Read the model definition and answer for the solid it produces. Units are mm, in the model's axes. Face numbers are marked on the shaded views. Give positions to 0.01 mm unless a question says otherwise; leave off trailing zeros. Write each loop counter-clockwise with the first axis right and the second up, starting at its lowest first coordinate (ties: lowest second). Pieces come first, ordered by that corner, then holes. Notation, with made-up numbers: (3.5, -33) - (42.5, -33) arc R32 cw to (42.5, -5) - close; hole circle Ø8 at (70, 21). An arc over 180 degrees is marked (long way). Answer as CSV lines item,"result".
Autodesk Inventor part; units mm, degrees
ref_plane "YZ Plane" through (0, 0, 0) normal (1, 0, 0) x (0, 1, 0)
ref_plane "XZ Plane" through (0, 0, 0) normal (0, 1, 0) x (-1, 0, 0)
ref_plane "XY Plane" through (0, 0, 0) normal (0, 0, 1) x (1, 0, 0)
sketch "Sketch1" plane through (0, 0, 0) normal (0, 1, 0) x (-1, 0, 0)
  circle A0 centre (1.143, 0) radius 39 construction
  circle A1 centre (1.143, 0) radius 42
  line L0 (-21.857, 14) -> (-36.857, 14) construction
  line L1 (-36.857, 14) -> (-36.857, 5) construction
  line L2 (-36.857, 5) -> (-21.857, 5) construction
  line L3 (-21.857, 5) -> (-21.857, 14) construction
  line L4 (1.143, 0) -> (-37.857, 0)
  line L5 (0, 0) -> (0, -22) construction
  dimension "d0" = 78
  dimension "d1" = 9
  dimension "d2" = 15
  dimension "d3" = 5
  dimension "d4" = 23
  dimension "d5" = 84
  dimension "d11" = 1.143
extrude "Extrusion1" add sketch "Sketch1" along normal blind 6
fillet "Fillet1" radius 7 1 edges at (40.857, 0, 0)
shell "Shell1" thickness 2 removed faces 1 at (-4.0377, 6, 12.235)
sketch "Sketch2" plane through (-1.143, 2, 0) normal (0, 1, 0) x (1, 0, 0)
  circle A0 centre (-11.303, -22.606) radius 1.95
  circle A1 centre (18.034, 6.223) radius 1.95
  circle A2 centre (-11.303, -22.606) radius 3.5
  circle A3 centre (18.034, 6.223) radius 3.5
  point P0 (1.143, 0)
  dimension "d12" = 3.9
  dimension "d13" = 3.9
  dimension "d14" = 6.223
  dimension "d15" = 16.891
  dimension "d16" = 22.606
  dimension "d17" = 12.446
  dimension "d18" = 7
  dimension "d19" = 7
extrude "Extrusion2" add sketch "Sketch2" along normal blind 5.5
sketch "Sketch3" plane through (-1.143, 2, 0) normal (0, 1, 0) x (1, 0, 0)
  line L0 (7.5, 19.5) -> (-25.5, 19.5) construction
  line L1 (-25.5, 19.5) -> (-25.5, -9.5) construction
  line L2 (-25.5, -9.5) -> (7.5, -9.5) construction
  line L3 (7.5, -9.5) -> (7.5, 19.5) construction
  line L4 (7.5, 19.5) -> (-25.5, -9.5) construction
  line L5 (-25.5, 19.5) -> (7.5, -9.5) construction
  point P0 (1.143, 0)
  point P1 (-9, 5)
  dimension "d22" = 33
  dimension "d23" = 29
sketch "Sketch5" plane through (-1.143, 6, 0) normal (0, 1, 0) x (1, 0, 0)
  line L0 (31.143, -15) -> (45, -15)
  line L1 (45, -15) -> (45, -3)
  line L2 (45, -3) -> (31.143, -3)
  line L3 (31.143, -3) -> (31.143, -15)
  line L4 (1.143, 0) -> (-32, 0) construction
  line L5 (31.143, 15) -> (45, 15)
  line L6 (45, 15) -> (45, 3)
  line L7 (45, 3) -> (31.143, 3)
  line L8 (31.143, 3) -> (31.143, 15)
  line L9 (-5.857, 30) -> (6.143, 30)
  line L10 (6.143, 30) -> (6.143, 46)
  line L11 (6.143, 46) -> (-5.857, 46)
  line L12 (-5.857, 46) -> (-5.857, 30)
  line L13 (-5.857, 30) -> (6.143, 46) construction
  line L14 (6.143, 30) -> (-5.857, 46) construction
  line L15 (-4.873, -22) -> (5.127, -22)
  line L16 (5.127, -22) -> (5.127, -44)
  line L17 (5.127, -44) -> (-4.873, -44)
  line L18 (-4.873, -44) -> (-4.873, -22)
  line L19 (-4.873, -22) -> (5.127, -44) construction
  line L20 (5.127, -22) -> (-4.873, -44) construction
  point P0 (0.143, 38)
  point P1 (0.127, -33)
  dimension "d24" = 3
  dimension "d25" = 12
  dimension "d26" = 30
  dimension "d29" = 1
  dimension "d30" = 12
  dimension "d31" = 1.016
  dimension "d32" = 10
extrude "Extrusion3" cut sketch "Sketch5" against normal up to surface (4 mm away)
mirror "Mirror1" about plane through (0, 0, 0) normal (0, 0, 1) of "Extrusion2"
sketch "Sketch6" plane through (-12.446, 7.5, 22.606) normal (0, 1, 0) x (1, 0, 0)
  circle A0 centre (0, 0) radius 4.9497
  circle A1 centre (29.337, 28.829) radius 1.95
  circle A2 centre (29.337, 28.829) radius 4.3979
  point P0 (12.446, 22.606)
extrude "Extrusion4" cut sketch "Sketch6" against normal up to surface (5.5 mm away) contours A0 | A1 | A2
properties part number "Case top"
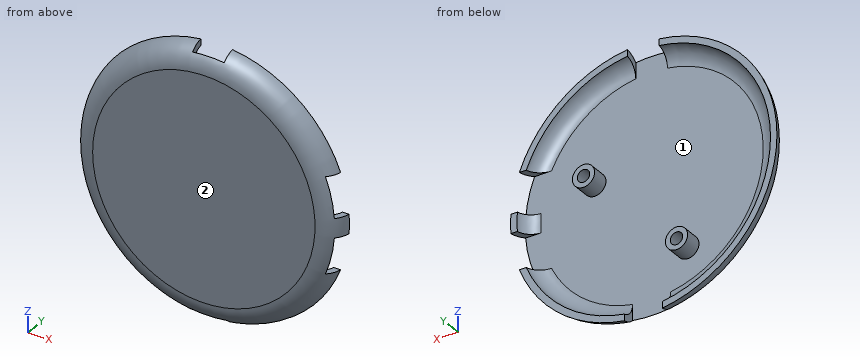
(1) A cutting plane is placed at A-A (y = 4). Write down the section's boundary in (x, z), and give its area (3 significant figures).
Worked out:
outline,"circle Ø7 at (-12.45, -22.61); (-7, -40.98) - (-7, -38.63) arc R39.07 cw to (-6.02, 38.77) - (-6.02, 41.11) arc R41.4 ccw to start; (3.98, 38.73) arc R39.07 cw to (34.93, 15) - (37.44, 15) arc R41.4 ccw to (3.98, 41.08) - close; (5, -40.94) arc R41.4 ccw to (37.44, -15) - (34.93, -15) arc R39.07 cw to (5, -38.59) - close; circle Ø7 at (16.89, 6.22); (37.81, -3) - (40.14, -3) arc R41.4 ccw to (40.14, 3) - (37.81, 3) arc R39.07 cw to start; hole circle Ø3.9 at (-12.45, -22.61); hole circle Ø3.9 at (16.89, 6.22)"
area,"532 mm^2"
(2) The mould has two halves that part along X. Classify the marked faces 1 and 2: +X half, -X half, draft (parallel to the pull), parting line (faces both ways), or undercut.
Worked out:
face 1,"undercut"
face 2,"draft"
(3) Find the intervals of material crossed by L1, parallel to X at y = 5, z = 4.5; L2, parallel to X at y = 3.5, z = -23; L3, parallel to Y at x = -15, z = -31, in increasing order.
Worked out:
L1,"x = -42.68 to -40.54, 13.84 to 15.98, 17.8 to 19.94"
L2,"x = -35.25 to -32.2, -15.92 to -14.36, -10.54 to -8.97, 29.91 to 32.96"
L3,"y = 0 to 2"
(4) Each of these flat-tipped pins is pushed along its axis until it touches: P1, Ø2, axis at x = 19.5, y = 3.5, coming from the -Z side; P2, Ø3, axis at y = 3.5, z = 36.5, coming from the -X side; P3, Ø6, axis at x = 16.891, z = 6.223, coming from the +Y side; P4, Ø3, axis at x = 33, y = 4, coming from the -Z side. Where does it stop, or does it pass through?
Worked out:
P1,"stops at z = -36.39"
P2,"stops at x = -23.14"
P3,"stops at y = 7.5"
P4,"stops at z = -25.71"
